Input: part model. Units: mm. Frame: model coordinates. Give positions to 0.01 mm unless a question says otherwise; leave off trailing zeros. Loops run counter-clockwise (first coordinate to the right, second up) from the corner with the lowest first, then second, coordinate; pieces in that order, holes last.
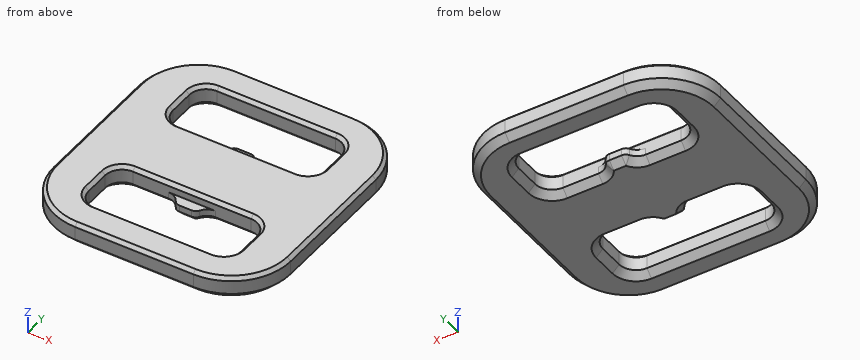
from build123d import *

# Parameters (mm, degrees)
F1_DEPTH = 7
F3_DEPTH = 4
F4_SIZE  = 1.99999
F8_SIZE  = 1


# Not quite as in the source:
# - a fillet or chamfer is up to 0.001 mm smaller than in the source, because OpenCascade refuses the exact size


with BuildPart() as f1:
    # F0 (on Top) → F1 (new body)
    with BuildSketch(Plane.XY):
        with BuildLine():
            Line((0, 10.5), (-17.5, 10.5))
            ThreePointArc((-17.5, 10.5), (-21.0355339059, 11.9644660941), (-22.5, 15.5))
            Line((-22.5, 15.5), (-22.5, 23))
            ThreePointArc((-22.5, 23), (-21.0355339059, 26.5355339059), (-17.5, 28))
            Line((-17.5, 28), (0, 28))
            Line((0, 28), (0, 37))
            Line((0, 37), (-17.5, 37))
            ThreePointArc((-17.5, 37), (-29.8743686708, 31.8743686708), (-35, 19.5))
            Line((-35, 19.5), (-35, 0))
            Line((-35, 0), (0, 0))
            Line((0, 0), (0, 10.5))
        make_face()
    extrude(amount=F1_DEPTH)

    # F2 (on Top) → F3 (join)
    with BuildSketch(Plane.XY):
        with BuildLine():
            Line((-7, 10.5), (0, 10.5))
            Line((0, 10.5), (0, 13.5))
            Line((0, 13.5), (-1.8038475773, 13.5))
            ThreePointArc((-1.8038475773, 13.5), (-2.8038475773, 13.2320508076), (-3.5358983849, 12.5))
            ThreePointArc((-3.5358983849, 12.5), (-5, 11.0358983849), (-7, 10.5))
        make_face()
    extrude(amount=F3_DEPTH)

    # F4 (size 2 in the source; OpenCascade refuses exactly that, so slightly less here)
    f4_edges = [f1.edges().sort_by_distance(p)[0] for p in [
        (-0.901924, 13.5, 0),
        (-35, 9.75, 0),
    ]]
    chamfer(f4_edges, length=F4_SIZE)

    # F6: F1 across face


with BuildPart() as f1_1:
    add(f1.part)
    add(f1.part.mirror(Plane(origin=(0, 6.0384247014, 3.3522948458), x_dir=(0, 1, 0), z_dir=(1, 0, 0))))

    # F7: F1 across face


with BuildPart() as f1_2:
    add(f1_1.part)
    add(f1_1.part.mirror(Plane(origin=(0, 0, 3.5233194082), x_dir=(1, 0, 0), z_dir=(0, -1, 0))))

    # F8
    f8_edges = [f1_2.edges().sort_by_distance(p)[0] for p in [
        (29.874369, 31.874369, 7),
        (0, 37, 7),
        (-29.874369, 31.874369, 7),
        (-35, 0, 7),
        (-29.874369, -31.874369, 7),
        (0, -37, 7),
        (29.874369, -31.874369, 7),
        (35, 0, 7),
        (-21.035534, 11.964466, 7),
        (-22.5, 19.25, 7),
        (-21.035534, 26.535534, 7),
        (0, 28, 7),
        (21.035534, 26.535534, 7),
        (22.5, 19.25, 7),
        (21.035534, 11.964466, 7),
        (0, 10.5, 7),
        (0, -10.5, 7),
        (21.035534, -11.964466, 7),
        (22.5, -19.25, 7),
        (21.035534, -26.535534, 7),
        (0, -28, 7),
        (-21.035534, -26.535534, 7),
        (-22.5, -19.25, 7),
        (-21.035534, -11.964466, 7),
    ]]
    chamfer(f8_edges, length=F8_SIZE)


solid = f1_2.part
(1) Cut plane A-A (x = -11). Return the cut outline in (y, z).
Values follow:
outline: (-37, 2) - (-35, 0) - (-30, 0) - (-28, 2) - (-28, 6) - (-29, 7) - (-36, 7) - (-37, 6) - close; (-10.5, 2) - (-8.5, 0) - (8.5, 0) - (10.5, 2) - (10.5, 6) - (9.5, 7) - (-9.5, 7) - (-10.5, 6) - close; (28, 2) - (30, 0) - (35, 0) - (37, 2) - (37, 6) - (36, 7) - (29, 7) - (28, 6) - close
(2) Cut plane B-B (z = 3). Count the separate pieces of the cut face and the enclosed holes in it, and give its area (3 significant figures).
Values follow:
separate pieces: 1
enclosed holes: 2
area: 3,430 mm2
(3) Pin query (flat end, axial travel): pin 1 Ø3 at (y, z) = (-28, 1.5) entering from -X; pin 2 Ø0.9 at (x, y) = (-3, -12.5) entering from +Z. Return the tip coordinate at first contact, or that it passes through.
Values follow:
pin 1: stops at x = -33.5
pin 2: stops at z = 4
(4) Ray query, probe 1 along Y at (x, z) = (-16, 3); probe 2 along Y at (x, z) = (9, 1); probe 3 along X at (y, z) = (-19.5, 5.5). Return the intervals inside material, ascending.
Values follow:
probe 1: y = -37 to -28, -10.5 to 10.5, 28 to 37
probe 2: y = -36 to -29, -9.5 to 9.5, 29 to 36
probe 3: x = -35 to -22.5, 22.5 to 35
